Design review of the part built by this model. Coordinates are the model's own, in mm. Face numbers are marked on the shaded views. A direction names the side the tool comes from. Round coordinates to 2 decimals unless told otherwise and drop trailing zeros. Order: outer loops, then holes, each group sorted by start corner. A loop starts at its lowest first (then second) coordinate and runs counter-clockwise, first axis right, second up. Notation, with made-up numbers: (32.25, 6) - (88.25, 6) arc R35 cw to (88.25, 39) - close; hole circle Ø6 at (19.5, 27). An arc over 180 degrees is marked (long way). Write item = value, one per line.
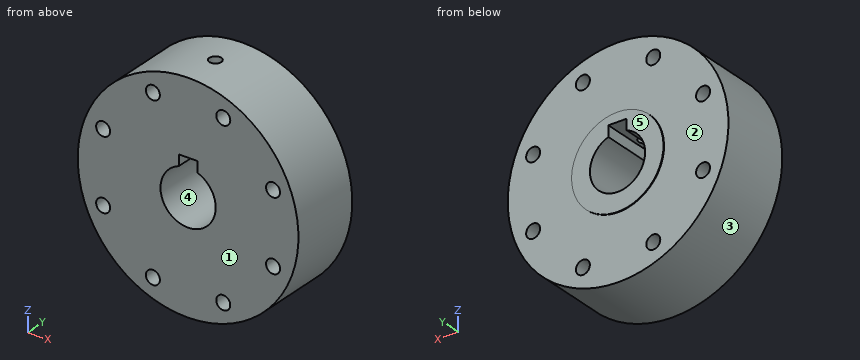
from build123d import *

# Parameters (mm, degrees)
SKETCH1_R              = 38.1
SKETCH1_R_2            = 9.525
BOSS_EXTRUDE1_DEPTH    = 25.4
F_10_32_TAPPED_HOLE1_D = 4.826
CIRPATTERN1_COUNT      = 8
SKETCH4_W              = 6.35
SKETCH4_H              = 6.35
CUT_EXTRUDE1_DEPTH     = 60.56828015
SKETCH5_W              = 2.0828
SKETCH5_H              = 25.4
SKETCH7_OUTSIDE_W      = 100.344
SKETCH7_OUTSIDE_H      = 100.344
SKETCH7_OUTSIDE_R      = 15.875
CUT_EXTRUDE2_DEPTH     = 0.254


with BuildPart() as part:
    # Sketch1 → Boss-Extrude1 (new body)
    with BuildSketch(Plane(origin=(0, 0, 0), x_dir=(1, 0, 0), z_dir=(0, 1, 0))):
        with Locations(Location((0, 0, 0), (0, 0, 270))):
            Circle(SKETCH1_R)
        with Locations(Location((0, 0, 0), (0, 0, 270))):
            Circle(SKETCH1_R_2, mode=Mode.SUBTRACT)
    extrude(amount=BOSS_EXTRUDE1_DEPTH)

    # #10-32 Tapped Hole1 (through all)
    with Locations(Plane(origin=(0, 25.4, 0), x_dir=(-1, 0, 0), z_dir=(0, 1, 0))):
        with Locations((29.333175157, -12.150198978)):
            f_10_32_tapped_hole1 = Hole(F_10_32_TAPPED_HOLE1_D / 2)

    # CirPattern1: #10-32 Tapped Hole1 ×8 about axis
    cirpattern1_axis = Axis((0, 0, 0), (0, 1, 0))
    for i in range(1, CIRPATTERN1_COUNT):
        add(f_10_32_tapped_hole1.rotate(cirpattern1_axis, i * 360 / CIRPATTERN1_COUNT), mode=Mode.SUBTRACT)

    # Sketch4 → Cut-Extrude1 (cut, through all)
    with BuildSketch(Plane(origin=(0, 25.4, 0), x_dir=(1, 0, 0), z_dir=(0, 1, 0))):
        with Locations((0, -9.525)):
            Rectangle(SKETCH4_W, SKETCH4_H)
    extrude(amount=-CUT_EXTRUDE1_DEPTH, mode=Mode.SUBTRACT)

    # Sketch5 → #8-32 Tapped Hole1 (revolve, cut)
    with BuildSketch(Plane(origin=(0, 12.7, 12.7), x_dir=(0, 1, 0), z_dir=(1, 0, 0))):
        with Locations((1.0414, 12.7)):
            Rectangle(SKETCH5_W, SKETCH5_H)
    revolve(axis=Axis((0, 12.7, 6.35), (0, 0, 1)), mode=Mode.SUBTRACT)

    # Sketch7 outside → Cut-Extrude2 (cut)
    with BuildSketch(Plane(origin=(0, 25.4, 0), x_dir=(1, 0, 0), z_dir=(0, 1, 0))):
        Rectangle(SKETCH7_OUTSIDE_W, SKETCH7_OUTSIDE_H)
        with Locations(Location((0, 0, 0), (0, 0, 270))):
            Circle(SKETCH7_OUTSIDE_R, mode=Mode.SUBTRACT)
    extrude(amount=-CUT_EXTRUDE2_DEPTH, mode=Mode.SUBTRACT)


solid = part.part
Item 1: Take a section at A-A, the plane x = 0. State the section outline as (y, z) points (3 decimals).
Data:
outline = (0, -38.1) - (25.146, -38.1) - (25.146, -15.875) - (25.4, -15.875) - (25.4, -9.525) - (0, -9.525) - close; (0, 12.7) - (10.617, 12.7) - (10.617, 38.1) - (0, 38.1) - close; (14.783, 12.7) - (25.4, 12.7) - (25.4, 15.875) - (25.146, 15.875) - (25.146, 38.1) - (14.783, 38.1) - close
Item 2: Take a section at B-B, the plane z = 0. State the section outline as (x, y) points (3 decimals).
Data:
outline = (-38.1, 0) - (-9.525, 0) - (-9.525, 25.4) - (-15.875, 25.4) - (-15.875, 25.146) - (-38.1, 25.146) - close; (9.525, 0) - (38.1, 0) - (38.1, 25.146) - (15.875, 25.146) - (15.875, 25.4) - (9.525, 25.4) - close
Item 3: For line 1 along Z through (x, y) = (11, 22); line 2 along X through (y, z) = (23, 31.5); line 3 along Z through (x, y) = (27.5, 19.25), list the stretches that pass through material, from the lowest coordinate up. Write a range as [from, to].
Data:
line_1 = [-36.48, -31.45], [-27.21, 27.21], [31.45, 36.48]
line_2 = [-21.43, -13.21], [-11.09, 11.09], [13.21, 21.43]
line_3 = [-26.37, -13.72], [-10.58, 10.58], [13.72, 26.37]
Item 4: Insertion check: P1, Ø5.5, axis at x = 29.33, z = -12.15, coming from the +Y side; P2, Ø6, axis at x = 14, y = 18.5, coming from the +Z side; P3, Ø4, axis at y = 3, z = -19, coming from the +X side. Each pin has a flat end and moves straight along its axis. Give the tip position at first contact, or say it passes through.
Data:
P1 = 25.15
P2 = 36.48
P3 = 34.1
Item 5: For the marked faces 1 and 2, list the 3-axis set-ups (+Z, -Z, +X, -X, +Y, -Y) from which the entire face can be reached by the end or side of a thin tool; tool diameter is ignored.
Data:
face_1 = +Z, -Z, +X, -X, -Y
face_2 = +Y
Item 6: The part is to be moulded in two halves that separate along X. For the marked faces 3, 4 and 5, say which applies: +X half, -X half, draft (parallel to the pull), parting line (faces both ways), or undercut.
Data:
face_3 = parting line
face_4 = undercut
face_5 = draft
Item 7: Take a section at C-C, the plane y = 20.25. Count the separate pieces of the cut face and the enclosed holes in it, and give its area (3 significant figures).
Data:
separate_pieces = 1
enclosed_holes = 9
area = 4,110 mm2
